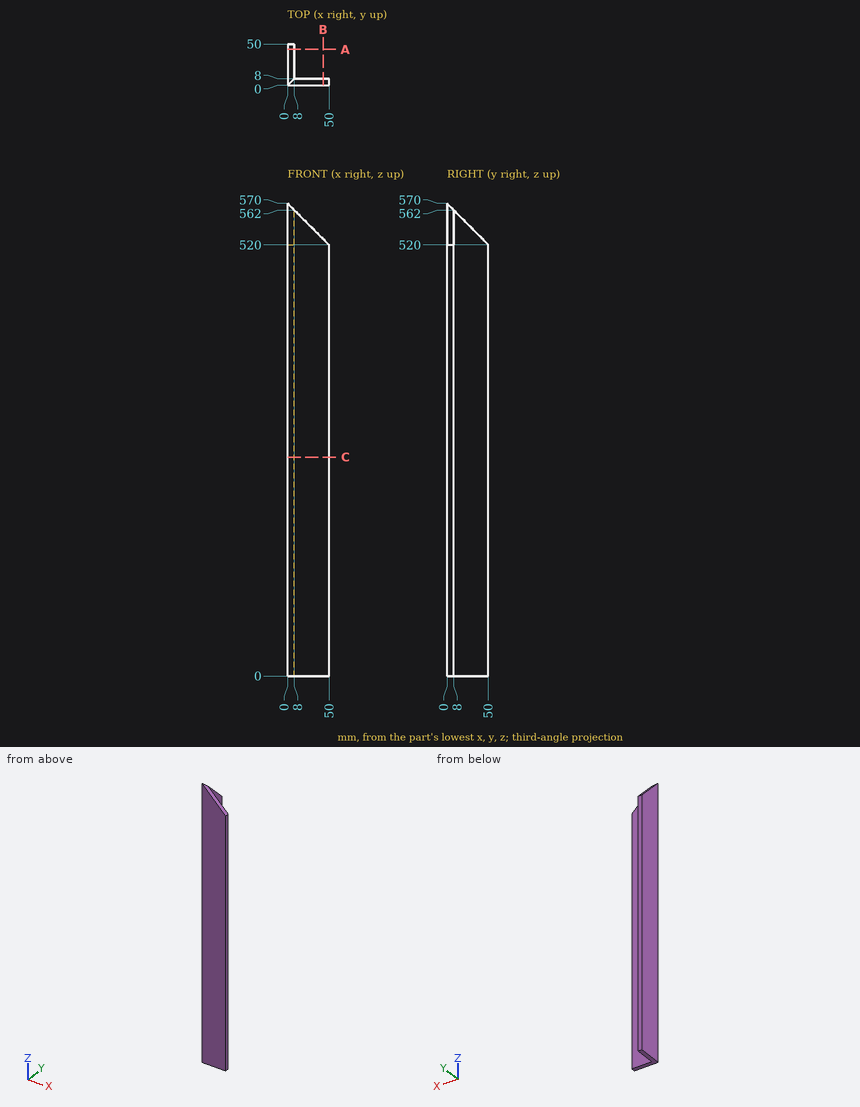
Geometry: see drawing. Coordinates: mm, zero at the bounding-box minimum. Give positions to 0.01 mm unless a question says otherwise; leave off trailing zeros. Order: outer loops, then holes, each group sorted by start corner. A loop starts at its lowest first (then second) coordinate and runs counter-clockwise, first axis right, second up. Notation, with made-up numbers: (57, 69.25) - (113, 69.25) arc R17 cw to (113, 86.25) - close; hole circle Ø9 at (67.25, 51). An arc over 180 degrees is marked (long way). Use CSV: the item, a comma, the result in double quotes.
1. Contact query for a flat-ended pin moving along its axis: pin 1 (2 mm diameter, centred on y = 12, z = 235, fed in from +X). Output: stop coordinate, or through.
Answers below:
pin 1,"x = 8"
2. Material intervals for line 1 along X through (y, z) = (17, 199); line 2 along Z through (x, y) = (5, 4.5), sorted ascending. Write a range as from..to.
Answers below:
line 1,"0..8"
line 2,"0..565"
3. Section query C-C (z = 264). Output: boundary loops of the cut face in (x, y).
Answers below:
outline,"(0, 0) - (50, 0) - (50, 8) - (8, 8) - (8, 50) - (0, 50) - close"
4. Section query A-A (y = 43.5). Output: boundary loops of the cut face in (x, z).
Answers below:
outline,"(0, 0) - (8, 0) - (8, 526.5) - (0, 526.5) - close"
5. Section query B-B (x = 43). Output: boundary loops of the cut face in (y, z), plus the area to 3 significant figures.
Answers below:
outline,"(0, 0) - (8, 0) - (8, 527) - (0, 527) - close"
area,"4,220 mm2"
